Work out the finished part from the listing and answer in its coordinate system (mm). A direction names the side the tool comes from. Round coordinates to 2 decimals unless told otherwise and drop trailing zeros. Loops run counter-clockwise (first coordinate to the right, second up) from the corner with the lowest first, then second, coordinate; pieces in that order, holes last. Notation, with made-up numbers: (-40, 25.25) -> (14, 25.25) arc R19 cw to (14, 33.25) -> close; hole circle Ø2 at (28, -38.5). An arc over 180 degrees is marked (long way). Write item = value, one per line. Start each with the question number.
```python
from build123d import *

# Parameters (mm, degrees)
SKETCH1_R           = 19.05
BOSS_EXTRUDE1_DEPTH = 38.1
CUT_EXTRUDE5_DEPTH  = 39.1
SKETCH8_W           = 184.15
SKETCH8_H           = 38.1127
CUT_EXTRUDE6_DEPTH  = 39.1
SKETCH9_W           = 88.9
SKETCH9_H           = 38.1
CUT_EXTRUDE7_DEPTH  = 39.1


with BuildPart() as part:
    # Sketch1 → Boss-Extrude1 (new body)
    with BuildSketch(Plane(origin=(0, 0, 0), x_dir=(1, 0, 0), z_dir=(0, 1, 0))):
        Polygon((0, 0), (774.7, 0), (774.7, -38.1), (863.6, -38.1), (863.6, -179.3875), (0, -179.3875), align=None)
        with Locations((627.126, -73.914)):
            Circle(SKETCH1_R, mode=Mode.SUBTRACT)
    extrude(amount=BOSS_EXTRUDE1_DEPTH)

    # Sketch7 → Cut-Extrude5 (cut, through all)
    with BuildSketch(Plane(origin=(0, 38.1, 0), x_dir=(1, 0, 0), z_dir=(0, 1, 0))):
        Polygon((455.6125, -141.2875), (487.3625, -141.2875), (487.3625, -122.2375), (544.5125, -122.2375), (544.5125, -179.3875), (455.6125, -179.3875), align=None)
    extrude(amount=-CUT_EXTRUDE5_DEPTH, mode=Mode.SUBTRACT)

    # Sketch8 → Cut-Extrude6 (cut, through all)
    with BuildSketch(Plane(origin=(0, 38.1, 0), x_dir=(1, 0, 0), z_dir=(0, 1, 0))):
        with Locations((771.525, -160.33115)):
            Rectangle(SKETCH8_W, SKETCH8_H)
    extrude(amount=-CUT_EXTRUDE6_DEPTH, mode=Mode.SUBTRACT)

    # Sketch9 → Cut-Extrude7 (cut, through all)
    with BuildSketch(Plane.XZ):
        with Locations((44.45, 19.05)):
            Rectangle(SKETCH9_W, SKETCH9_H)
    extrude(amount=-CUT_EXTRUDE7_DEPTH, mode=Mode.SUBTRACT)


solid = part.part
```
Item 1: Flat-ended cylindrical pins translate along their axes: pin 1 (19 mm diameter, centred on y = 28, z = 16.5, fed in from -X); pin 2 (19 mm diameter, centred on x = 41, y = 11, fed in from -Z); pin 3 (11.5 mm diameter, centred on y = 22.5, z = 169, fed in from +X). Find the tip coordinate at first contact, or state that the pin passes through.
Item 2: Section D-D (z = 84) is taken. Determine the outline of the cut face in (x, y).
Item 3: Find the intervals of material crossed by line 1 along X through (y, z) = (3, 74); line 2 along X through (y, z) = (19, 163); line 3 along X through (y, z) = (17, 26.5), in increasing order. Write a range as [from, to].
Item 4: Section B-B (y = 23.5) is taken. Determine the outline of the cut face in (x, z), then the cut area to 3 significant figures.
Item 5: Section C-C (x = 474.5) is taken. Determine the outline of the cut face in (y, z), then the cut area to 3 significant figures.
Item 6: A tool of negligible diameter and unlimited length cuts with its end or side. For faces 4 (the flat face through (819, 19, 38.1)), 5 (the flat face through (471, 19, 141.288)), 6 (the flat face through (770, 19, 141.275)), 7 (the flat face through (613, 19, 179.388)), 8 (the flat face through (863.6, 19, 89)), from which of +Z, -Z, +X, -X, +Y, -Y can it reach the whole face along a straight path? Write none if from no direction.
Item 7: Section A-A (z = 151) is taken. Determine the outline of the cut face in (x, y), then the cut area to 3 significant figures.
Item 8: The mould has two halves that part along X. Classify faces 1 (the flat face through (487.362, 19, 132)), 2 (the flat face through (44, 19, 38.1)), 3 (the flat face through (88.9, 19, 19)): pulls with the +X half, pulls with the -X half, needs draft (parallel to the pull), parting line crosses it, or undercut.
Worked answers:
q1.pin_1 = 88.9
q1.pin_2 = 38.1
q1.pin_3 = 679.45
q2.outline = (0, 0) -> (610.97, 0) -> (610.97, 38.1) -> (0, 38.1) -> close; (643.29, 0) -> (863.6, 0) -> (863.6, 38.1) -> (643.29, 38.1) -> close
q3.line_1 = [0, 608.08], [646.18, 863.6]
q3.line_2 = [0, 455.61], [544.51, 679.45]
q3.line_3 = [88.9, 774.7]
q4.outline = (0, 38.1) -> (88.9, 38.1) -> (88.9, 0) -> (774.7, 0) -> (774.7, 38.1) -> (863.6, 38.1) -> (863.6, 141.27) -> (679.45, 141.27) -> (679.45, 179.39) -> (544.51, 179.39) -> (544.51, 122.24) -> (487.36, 122.24) -> (487.36, 141.29) -> (455.61, 141.29) -> (455.61, 179.39) -> (0, 179.39) -> close; hole circle Ø38.1 at (627.13, 73.91)
q4.area = 136,000 mm2
q5.outline = (0, 0) -> (38.1, 0) -> (38.1, 141.29) -> (0, 141.29) -> close
q5.area = 5,380 mm2
q6.face_4 = -Z, +X, +Y, -Y
q6.face_5 = +Z, +Y, -Y
q6.face_6 = +Z, +X, +Y, -Y
q6.face_7 = +Z, +X, -X, +Y, -Y
q6.face_8 = +Z, -Z, +X, +Y, -Y
q7.outline = (0, 0) -> (455.61, 0) -> (455.61, 38.1) -> (0, 38.1) -> close; (544.51, 0) -> (679.45, 0) -> (679.45, 38.1) -> (544.51, 38.1) -> close
q7.area = 22,500 mm2
q8.face_1 = undercut
q8.face_2 = needs draft
q8.face_3 = pulls with the -X half
